```python
from build123d import *

# Parameters (mm, degrees)
CUT_EXTRUDE_START   = -20
CUT_EXTRUDE_1_DEPTH = 20


with BuildPart() as part:
    # 草图1 → 旋转1 (revolve)
    with BuildSketch(Plane.XY, mode=Mode.PRIVATE) as revolve_1_sk:
        Polygon((0, 2), (1.5, 2), (1.5, 0), (11, 0), (11, 1.5), (9.2, 1.5), (9.2, 4), (11, 4), (11, 5.5), (9.2, 5.5), (9.2, 8), (11, 8), (11, 9.5), (9.2, 9.5), (9.2, 12), (11, 12), (11, 13.5), (9.2, 13.5), (9.2, 16), (13, 16), (13, -1.584568421), (0, -1.584568421), (0, 0), align=None)
    revolve(revolve_1_sk.sketch.rotate(Axis((0, 18, 0), (0, -1, 0)), 180), axis=Axis((0, 18, 0), (0, -1, 0)))

    # 草图2 → 切除-拉伸1 (cut)
    with BuildSketch(Plane(origin=(0, 16, 0), x_dir=(1, 0, 0), z_dir=(0, 1, 0)).offset(CUT_EXTRUDE_START)):
        with BuildLine():
            Line((-13, 0), (13, 0))
            ThreePointArc((13, 0), (0, 13), (-13, 0))
        make_face()
    extrude(amount=CUT_EXTRUDE_1_DEPTH, mode=Mode.SUBTRACT)


solid = part.part
```
CAD build for the part. Positions are in the model's coordinates, mm. A direction names the side the tool comes from. Coordinates: 2 decimals unless noted, no trailing zeros. Loops run counter-clockwise (first coordinate to the right, second up) from the corner with the lowest first, then second, coordinate; pieces in that order, holes last. Notation, with made-up numbers: (52.5, 28.5) - (95.5, 28.5) arc R25 ccw to (95.5, 60.5) - close; hole circle Ø5 at (21, 40). An arc over 180 degrees is marked (long way). Return JSON: item names as keys, results as strings.
1. Probe L1, parallel to Y at x = -1.75, z = 9.5; L2, parallel to Z at x = -5, y = -0.25; L3, parallel to Y at x = 0.25, z = 1.75. List the from-to ranges inside material, lowest first. Write a range as from..to.
Result:
{"L1": "y = -1.58..0, 1.5..4, 5.5..8, 9.5..12, 13.5..16", "L2": "z = 0..12", "L3": "y = -1.58..0"}
2. Band-saw the part on C-C (y = 3.25). Give the cut face in (x, z), and give its area (3 significant figures).
Result:
{"outline": "(-13, 0) - (-9.2, 0) arc R9.2 cw to (9.2, 0) - (13, 0) arc R13 ccw to start", "area": "133 mm2"}
3. 3-axis set-ups, long thin cutter, end or side, ignore diameter. For faces 1 (the cylindrical face through (0.202, 6.768, 9.198)), 2 (the flat face through (0, 1, 0)), 3 (the flat face through (-2, 12, 10)): which of +Z, -Z, +X, -X, +Y, -Y reach the whole face in a straight line?
Result:
{"face 1": "-Z, +Y", "face 2": "-Z, +X, -X, +Y, -Y", "face 3": "-Z"}
4. Band-saw the part on B-B (x = 0). Give the cut face in (y, z).
Result:
{"outline": "(-1.58, 0) - (2, 0) - (2, 1.5) - (0, 1.5) - (0, 11) - (1.5, 11) - (1.5, 9.2) - (4, 9.2) - (4, 11) - (5.5, 11) - (5.5, 9.2) - (8, 9.2) - (8, 11) - (9.5, 11) - (9.5, 9.2) - (12, 9.2) - (12, 11) - (13.5, 11) - (13.5, 9.2) - (16, 9.2) - (16, 13) - (-1.58, 13) - close"}
5. Drop flat-ended pins along their axis: pin 1 (4 mm diameter, centred on x = 4, z = 4.5, fed in from +Y); pin 2 (6 mm diameter, centred on x = 4, y = 5, fed in from -Z); pin 3 (1 mm diameter, centred on x = -9, y = 0.5, fed in from +Z). Give the stop position or say it passes through.
Result:
{"pin 1": "stops at y = 0", "pin 2": "stops at z = 6.02", "pin 3": "stops at z = 9.84"}
6. Band-saw the part on A-A (z = 10.5). Give the cut face in (x, y), and give its area (3 significant figures).
Result:
{"outline": "(-7.66, -1.58) - (7.66, -1.58) - (7.66, 16) - (-7.66, 16) - close; hole (-3.28, 0) - (3.28, 0) - (3.28, 1.5) - (-3.28, 1.5) - close; hole (-3.28, 4) - (3.28, 4) - (3.28, 5.5) - (-3.28, 5.5) - close; hole (-3.28, 8) - (3.28, 8) - (3.28, 9.5) - (-3.28, 9.5) - close; hole (-3.28, 12) - (3.28, 12) - (3.28, 13.5) - (-3.28, 13.5) - close", "area": "230 mm2"}
7. Band-saw the part on D-D (x = -10.5). Give the cut face in (y, z).
Result:
{"outline": "(-1.58, 0) - (0, 0) - (0, 3.28) - (1.5, 3.28) - (1.5, 0) - (4, 0) - (4, 3.28) - (5.5, 3.28) - (5.5, 0) - (8, 0) - (8, 3.28) - (9.5, 3.28) - (9.5, 0) - (12, 0) - (12, 3.28) - (13.5, 3.28) - (13.5, 0) - (16, 0) - (16, 7.66) - (-1.58, 7.66) - close"}
8. Mould opens along Z. For faces 4 (the flat face through (0, 0, 4)), 5 (the cylindrical face through (0.202, 14.768, 9.198)), 6 (the flat face through (-2, 8, 10)) say: released by +Z, released by -Z, zero draft, split by the parting line, or undercut.
Result:
{"face 4": "undercut", "face 5": "released by -Z", "face 6": "zero draft"}
